```python
from build123d import *

# Parameters (mm, degrees)
SKETCH1_W                 = 100
SKETCH1_H                 = 15
BOSS_EXTRUDE1_DEPTH       = 5
SKETCH2_W                 = 5
SKETCH2_H                 = 15
BOSS_EXTRUDE2_DEPTH       = 45
SKETCH3_W                 = 55.52
SKETCH3_H                 = 5
BOSS_EXTRUDE3_DEPTH       = 5
F_5_0MM_DOWEL_SLOT1_DEPTH = 5
F_5_0MM_DOWEL_SLOT2_DEPTH = 5
F_5_0MM_DOWEL_HOLE1_D     = 5
F_5_0MM_DOWEL_HOLE2_D     = 5
BOSS_EXTRUDE4_DEPTH       = 5
BOSS_EXTRUDE5_DEPTH       = 5


# Read off the part's stored shape, not the designer's step: Ø5.0mm Dowel Slot1, Ø5.0mm Dowel Slot2
with BuildPart() as part:
    # Sketch1 → Boss-Extrude1 (new body)
    with BuildSketch(Plane(origin=(0, 0, 0), x_dir=(1, 0, 0), z_dir=(0, 1, 0))):
        with Locations((-3.34119197, 9.533232324)):
            Rectangle(SKETCH1_W, SKETCH1_H)
    extrude(amount=BOSS_EXTRUDE1_DEPTH)

    # Sketch2 → Boss-Extrude2 (add)
    with BuildSketch(Plane(origin=(0, 5, 0), x_dir=(1, 0, 0), z_dir=(0, 1, 0))):
        with Locations((-50.84119197, 9.533232324)):
            Rectangle(SKETCH2_W, SKETCH2_H)
    extrude(amount=BOSS_EXTRUDE2_DEPTH)

    # Sketch3 → Boss-Extrude3 (add)
    with BuildSketch(Plane(origin=(0, 0, 0), x_dir=(-1, 0, 0), z_dir=(0, -1, 0))):
        with Locations((-18.89880803, 19.533232324)):
            Rectangle(SKETCH3_W, SKETCH3_H)
        with Locations((-18.89880803, -0.466767676)):
            Rectangle(SKETCH3_W, SKETCH3_H)
    extrude(amount=-BOSS_EXTRUDE3_DEPTH)

    # Ø5.0mm Dowel Slot1 outline → Ø5.0mm Dowel Slot1 (cut)
    with BuildSketch(Plane(origin=(0, 0, 0), x_dir=(1, 0, 0), z_dir=(0, 1, 0))):
        with BuildLine():
            Line((44.842812818, 6.659177942), (44.842812818, 12.359177942))
            ThreePointArc((44.842812818, 12.359177942), (42.342812818, 14.859177942), (39.842812818, 12.359177942))
            Line((39.842812818, 12.359177942), (39.842812818, 6.659177942))
            ThreePointArc((39.842812818, 6.659177942), (42.342812818, 4.159177942), (44.842812818, 6.659177942))
        make_face()
    extrude(amount=F_5_0MM_DOWEL_SLOT1_DEPTH, mode=Mode.SUBTRACT)

    # Ø5.0mm Dowel Slot2 outline → Ø5.0mm Dowel Slot2 (cut)
    with BuildSketch(Plane(origin=(0, 0, 0), x_dir=(1, 0, 0), z_dir=(0, 1, 0))):
        with BuildLine():
            ThreePointArc((37.654614979, 12.36475158), (35.154614979, 14.86475158), (32.654614979, 12.36475158))
            Line((32.654614979, 12.36475158), (32.654614979, 6.66475158))
            ThreePointArc((32.654614979, 6.66475158), (35.154614979, 4.16475158), (37.654614979, 6.66475158))
            Line((37.654614979, 6.66475158), (37.654614979, 12.36475158))
        make_face()
    extrude(amount=F_5_0MM_DOWEL_SLOT2_DEPTH, mode=Mode.SUBTRACT)

    # Ø5.0mm Dowel Hole1 (through all)
    with Locations(Plane.ZY.offset(53.34119197)):
        with Locations((-9.533232324, 40), (-9.958577789, 15)):
            Hole(F_5_0MM_DOWEL_HOLE1_D / 2)

    # Ø5.0mm Dowel Hole2 (through all)
    with Locations(Plane(origin=(0, 5, 0), x_dir=(1, 0, 0), z_dir=(0, 1, 0))):
        with Locations((18.89880803, 9.533232324)):
            Hole(F_5_0MM_DOWEL_HOLE2_D / 2)

    # Sketch15 → Boss-Extrude4 (add)
    with BuildSketch(Plane.XY.offset(-2.033232324)):
        Polygon((-48.34119197, 50), (-8.86119197, 5), (-8.86119197, 0), (-53.34119197, 0), (-53.34119197, 50), align=None)
    extrude(amount=BOSS_EXTRUDE4_DEPTH)

    # Sketch16 → Boss-Extrude5 (add)
    with BuildSketch(Plane(origin=(0, 0, -17.033232324), x_dir=(-1, 0, 0), z_dir=(0, 0, -1))):
        Polygon((48.34119197, 50), (8.86119197, 5), (8.86119197, 0), (53.34119197, 0), (53.34119197, 50), align=None)
    extrude(amount=BOSS_EXTRUDE5_DEPTH)


solid = part.part
```
The listing builds one solid part. Answer for the finished solid, in the listing's coordinates (mm). A direction names the side the tool comes from. Give positions to 0.01 mm unless a question says otherwise; leave off trailing zeros. Order: outer loops, then holes, each group sorted by start corner. A loop starts at its lowest first (then second) coordinate and runs counter-clockwise, first axis right, second up. Notation, with made-up numbers: (-34.75, -11.75) -> (-11.75, -11.75) arc R23 cw to (-11.75, 15.25) -> close; hole circle Ø4 at (23.5, -23). An arc over 180 degrees is marked (long way). Answer as a JSON object with one key per item and string values. Group by question number.
Item 1: Flat-ended cylindrical pins translate along their axes: pin 1 (1 mm diameter, centred on x = -24.5, z = -3, fed in from +Y); pin 2 (5 mm diameter, centred on x = 20, y = 8.5, fed in from -Z); pin 3 (8 mm diameter, centred on y = 15, z = -9.96, fed in from +X). Find the tip coordinate at first contact, or state that the pin passes through.
Item 2: The part is cut by section C-C on y = 22. Write down the section's boundary in (x, z), and give its area (3 significant figures).
Item 3: The part is cut by section D-D on y = 4. Write down the section's boundary in (x, z), and give its area (3 significant figures).
Item 4: A tool of negligible diameter and unlimited length cuts with its end or side. For faces 1 (the flat face through (-37, 18, -17.033)), 2 (the flat face through (-25, 18, 2.967)), 3 (the flat face through (32.655, 2, -10)), from which of +Z, -Z, +X, -X, +Y, -Y can it reach the whole face along a straight path? Write none if from no direction.
Item 5: The part is cut by section A-A on y = 14. Write down the section's boundary in (x, z), and give its area (3 significant figures).
Item 6: Determine the mould class of faces 4 (the flat face through (0, 5, -10)), 5 (the cylindrical face through (35.21, 2.465, -14.864)), 6 (the cylindrical face through (-50.806, 14.042, -12.268)) for opening direction Y: pulls with the +Y half, pulls with the -Y half, needs draft (parallel to the pull), parting line crosses it, or undercut.
Item 7: Consider L1, parallel to Z at x = -39, y = 9; L2, parallel to X at y = 27.5, z = -17; L3, parallel to Y at x = 1, z = -15.5. Determine where each line is inside the solid, lowest interval first. Write a range as from..to.
Item 8: The part is cut by section B-B on z = -5.5. Write down the section's boundary in (x, y), and give its area (3 significant figures).
Result set:
{
 "1": {"pin 1": "y = 5", "pin 2": "through", "pin 3": "x = -48.34"},
 "2": {"outline": "(-53.34, -22.03) -> (-23.78, -22.03) -> (-23.78, -17.03) -> (-48.34, -17.03) -> (-48.34, -2.03) -> (-23.78, -2.03) -> (-23.78, 2.97) -> (-53.34, 2.97) -> close", "area": "371 mm²"},
 "3": {"outline": "(-53.34, -22.03) -> (46.66, -22.03) -> (46.66, 2.97) -> (-53.34, 2.97) -> close; hole circle Ø5 at (18.9, -9.53); hole (32.65, -12.36) arc R2.5 ccw to (37.65, -12.36) -> (37.65, -6.66) arc R2.5 ccw to (32.65, -6.66) -> close; hole (39.84, -12.36) arc R2.5 ccw to (44.84, -12.36) -> (44.84, -6.66) arc R2.5 ccw to (39.84, -6.66) -> close", "area": "2,380 mm²"},
 "4": {"face 1": "+X, +Y", "face 2": "+Z, +X, -X, +Y, -Y", "face 3": "+Y, -Y"},
 "5": {"outline": "(-53.34, -22.03) -> (-16.76, -22.03) -> (-16.76, -17.03) -> (-48.34, -17.03) -> (-48.34, -12.25) -> (-53.34, -12.25) -> close; (-53.34, -7.67) -> (-48.34, -7.67) -> (-48.34, -2.03) -> (-16.76, -2.03) -> (-16.76, 2.97) -> (-53.34, 2.97) -> close", "area": "418 mm²"},
 "6": {"face 4": "pulls with the +Y half", "face 5": "needs draft", "face 6": "undercut"},
 "7": {"L1": "-22.03..-17.03, -2.03..2.97", "L2": "-53.34..-48.34", "L3": "0..5"},
 "8": {"outline": "(-53.34, 0) -> (32.94, 0) -> (32.94, 5) -> (-48.34, 5) -> (-48.34, 50) -> (-53.34, 50) -> close; (37.37, 0) -> (40.13, 0) -> (40.13, 5) -> (37.37, 5) -> close; (44.56, 0) -> (46.66, 0) -> (46.66, 5) -> (44.56, 5) -> close", "area": "681 mm²"}
}
